Input: part model. Units: mm. Frame: model coordinates. A direction names the side the tool comes from. Round coordinates to 2 decimals unless told otherwise and drop trailing zeros. Loops run counter-clockwise (first coordinate to the right, second up) from the corner with the lowest first, then second, coordinate; pieces in that order, holes last. Notation, with made-up numbers: M 43.25,-12 L 61.25,-12 A23 cw 61.25,11 Z; hole C 4,11.5 d2. An arc over 180 degrees is marked long. Put each result on its own line as item: value. Start each with the question number.
1) Draft query along Z for faces 1 (the face through (-26, 46, 24.4)), 2 (the face through (-40.5, 28, 16)), 3 (the face through (-35, 28, 2)). Return one class per face: +Z half, -Z half, draft (parallel to the pull), parting line (faces both ways), or undercut.
2) Section B-B on x = -34. Output: boundary loops of the cut face in (y, z), plus the area to 3 significant figures.
3) Pin query (flat end, axial travel): pin 1 (2 mm diameter, centred on y = 39.5, z = 22, fed in from +X); pin 2 (14 mm diameter, centred on x = -18, z = 18, fed in from +Y); pin 3 (5 mm diameter, centred on x = -13, z = 19.5, fed in from +Y). Return the tip coordinate at first contact, or that it passes through.
4) Section D-D on x = -2. Output: boundary loops of the cut face in (y, z), plus the area to 4 significant figures.
5) Line query: probe 1 along Z at (x, y) = (-33, 17); probe 2 along Z at (x, y) = (-16, 53.7); probe 3 along X at (y, z) = (54.5, 16). Output: solid intervals per line, ascending.
6) Section A-A on z = 16. Output: boundary loops of the cut face in (x, y), plus the area to 3 significant figures.
7) Reachability of faces 4 (the face through (1.5, 27, 21)), 5 (the face through (-16, 31, 28)), 6 (the face through (-11.155, 54.014, 25.315)), 7 (the face through (-35, 27, 4)) from +Z, -Z, +X, -X, +Y, -Y: full face, straight path, thin tool, end or side. Return the list, or none.
8) Section C-C on y = 27.5. Output: boundary loops of the cut face in (x, z).
Autodesk Inventor part; units mm, degrees
ref_plane "YZ Plane" through (0, 0, 0) normal (1, 0, 0) x (0, 1, 0)
ref_plane "XZ Plane" through (0, 0, 0) normal (0, 1, 0) x (-1, 0, 0)
ref_plane "XY Plane" through (0, 0, 0) normal (0, 0, 1) x (1, 0, 0)
sketch "Sketch1" plane through (0, 0, 0) normal (0, 1, 0) x (-1, 0, 0)
  line L0 (32, 32) -> (0, 32)
  line L1 (0, 32) -> (0, 0)
  line L2 (0, 0) -> (32, 0)
  line L3 (32, 0) -> (32, 32)
extrude "Extrusion1" add sketch "Sketch1" along normal blind 55
sketch "Sketch2" plane through (0, 55, 0) normal (0, 1, 0) x (1, 0, 0)
  line L0 (-9.6, -9.6) -> (-22.4, -9.6)
  line L1 (-22.4, -9.6) -> (-22.4, -22.4)
  line L2 (-22.4, -22.4) -> (-9.6, -22.4)
  line L3 (-9.6, -22.4) -> (-9.6, -9.6)
  point P0 (0, 0)
extrude "Extrusion2" cut sketch "Sketch2" against normal blind 30
sketch "Sketch3" plane through (-32, 0, 32) normal (0, 0, 1) x (1, 0, 0)
  line L0 (3.5, 49) -> (28.5, 49)
  line L1 (28.5, 49) -> (28.5, 31)
  line L2 (28.5, 31) -> (3.5, 31)
  line L3 (3.5, 31) -> (3.5, 49)
  line L4 (3.5, 49) -> (3.5, 43.25)
  line L5 (3.5, 36.75) -> (3.5, 43.25)
  line L6 (28.5, 49) -> (28.5, 43.25)
  line L7 (28.5, 36.75) -> (28.5, 43.25)
  line L8 (3.5, 43.25) -> (3.5, 36.75)
  line L9 (28.5, 43.25) -> (28.5, 36.75)
  point P0 (32, 0)
extrude "Extrusion3" cut sketch "Sketch3" against normal blind 8.6
sketch "Sketch4" plane through (-32, 0, 23.4) normal (0, 0, 1) x (1, 0, 0)
  line L0 (3.5, 49) -> (28.5, 49)
  line L1 (3.5, 49) -> (3.5, 43.25)
  line L2 (28.5, 31) -> (3.5, 31)
  line L3 (3.5, 36.75) -> (3.5, 31)
  line L4 (3.5, 31) -> (28.5, 31)
  line L5 (28.5, 31) -> (28.5, 36.75)
  line L6 (28.5, 49) -> (28.5, 31)
  line L7 (28.5, 43.25) -> (28.5, 49)
  line L8 (28.5, 49) -> (3.5, 49)
  point P0 (32, 0)
sketch "Sketch5" plane through (-32, 0, 23.4) normal (0, 0, 1) x (1, 0, 0)
  line L0 (3.5, 43.25) -> (8.5, 43.25)
  line L1 (8.5, 43.25) -> (8.5, 36.75)
  line L2 (8.5, 36.75) -> (3.5, 36.75)
  line L3 (3.5, 36.75) -> (3.5, 43.25)
  point P0 (32, 0)
sketch "Sketch6" plane through (-32, 0, 23.4) normal (0, 0, 1) x (1, 0, 0)
  line L0 (28.5, 43.25) -> (23.5, 43.25)
  line L1 (23.5, 43.25) -> (23.5, 36.75)
  line L2 (23.5, 36.75) -> (28.5, 36.75)
  line L3 (28.5, 36.75) -> (28.5, 43.25)
  point P0 (32, 0)
extrude "Extrusion4" cut sketch "Sketch5" against normal blind 2
extrude "Extrusion5" cut sketch "Sketch6" against normal blind 2
sketch "Sketch7" plane through (-32, 0, 23.4) normal (0, 0, 1) x (1, 0, 0)
  line L0 (3.5, 43.25) -> (8.5, 43.25)
  line L1 (3.5, 43.25) -> (3.5, 49)
  line L2 (8.5, 43.25) -> (3.5, 43.25)
  line L3 (3.5, 43.25) -> (3.5, 49)
  line L4 (3.5, 49) -> (8.5, 49)
  line L5 (8.5, 49) -> (8.5, 43.25)
  point P0 (32, 0)
sketch "Sketch8" plane through (-32, 0, 23.4) normal (0, 0, 1) x (1, 0, 0)
  line L0 (8.5, 36.75) -> (3.5, 36.75)
  line L1 (28.5, 31) -> (3.5, 31)
  line L2 (8.5, 36.75) -> (3.5, 36.75)
  line L3 (3.5, 36.75) -> (3.5, 31)
  line L4 (3.5, 31) -> (8.5, 31)
  line L5 (8.5, 31) -> (8.5, 36.75)
  point P0 (32, 0)
sketch "Sketch9" plane through (-32, 0, 23.4) normal (0, 0, 1) x (1, 0, 0)
  line L0 (28.5, 36.75) -> (23.5, 36.75)
  line L1 (28.5, 31) -> (3.5, 31)
  line L2 (23.5, 36.75) -> (28.5, 36.75)
  line L3 (28.5, 36.75) -> (28.5, 31)
  line L4 (28.5, 31) -> (23.5, 31)
  line L5 (23.5, 31) -> (23.5, 36.75)
  point P0 (32, 0)
sketch "Sketch10" plane through (-32, 0, 23.4) normal (0, 0, 1) x (1, 0, 0)
  line L0 (23.5, 43.25) -> (28.5, 43.25)
  line L1 (28.5, 49) -> (28.5, 43.25)
  line L2 (23.5, 43.25) -> (28.5, 43.25)
  line L3 (28.5, 43.25) -> (28.5, 49)
  line L4 (28.5, 49) -> (23.5, 49)
  line L5 (23.5, 49) -> (23.5, 43.25)
  point P0 (32, 0)
extrude "Extrusion6" add sketch "Sketch7" along normal blind 1
extrude "Extrusion7" add sketch "Sketch8" along normal blind 1
extrude "Extrusion8" add sketch "Sketch9" along normal blind 1
extrude "Extrusion9" add sketch "Sketch10" along normal blind 1
sketch "Sketch11" plane through (-32, 0, 24.4) normal (0, 0, 1) x (1, 0, 0)
  line L0 (23.5, 43.25) -> (28.5, 43.25)
  line L1 (23.5, 43.25) -> (25, 43.25)
  line L2 (25, 43.25) -> (25, 44.25)
  line L3 (25, 44.25) -> (23.5, 44.25)
  line L4 (23.5, 44.25) -> (23.5, 43.25)
  point P0 (32, 0)
extrude "Extrusion10" cut sketch "Sketch11" against normal blind 1
sketch "Sketch12" plane through (-32, 0, 23.4) normal (0, 0, 1) x (1, 0, 0)
  line L0 (8.5, 49) -> (8.5, 43.25)
  line L1 (23.5, 31) -> (8.5, 31)
  line L2 (23.5, 49) -> (23.5, 44.25)
  point P0 (32, 0)
sketch "Sketch13" plane through (-32, 0, 23.4) normal (0, 0, 1) x (1, 0, 0)
  point P0 (32, 0)
sketch "Sketch14" plane through (-32, 0, 23.4) normal (0, 0, 1) x (1, 0, 0)
  line L0 (23.5, 44.25) -> (23.5, 49)
  line L1 (23.5, 49) -> (17.5, 49)
  line L2 (14.5, 43) -> (17.5, 43)
  line L3 (17.5, 38) -> (18, 38)
  line L4 (18, 38) -> (18, 43)
  line L5 (18, 43) -> (14, 43)
  line L6 (14, 43) -> (14, 38)
  line L7 (14, 38) -> (14.5, 38)
  line L8 (14.5, 38) -> (14.5, 42)
  line L9 (3.5, 43.25) -> (8.5, 43.25)
  line L10 (14.5, 42) -> (14.5, 42.5)
  line L11 (14.5, 42.5) -> (17.5, 42.5)
  line L12 (17.5, 42.5) -> (17.5, 38)
  point P0 (32, 0)
extrude "Extrusion11" add sketch "Sketch14" along normal blind 1
sketch "Sketch15" plane through (-32, 0, 23.4) normal (0, 0, 1) x (1, 0, 0)
  line L0 (14.5, 42.5) -> (14.5, 38)
  line L1 (14.5, 42.5) -> (17.5, 42.5)
  line L2 (17.5, 42.5) -> (17.5, 39.5)
  line L3 (17.5, 39.5) -> (14.5, 39.5)
  line L4 (14.5, 39.5) -> (14.5, 42.5)
  point P0 (32, 0)
extrude "Extrusion12" cut sketch "Sketch15" against normal blind 7.1
sketch "Sketch16" plane through (-32, 0, 32) normal (0, 0, 1) x (1, 0, 0)
  point P0 (32, 0)
sketch "Sketch17" plane through (0, 0, 32) normal (1, 0, 0) x (0, 0, -1)
  line L0 (2, 46) -> (20, 46)
  line L1 (20, 46) -> (20, 8)
  line L2 (20, 8) -> (2, 8)
  line L3 (2, 8) -> (2, 46)
  point P0 (32, 0)
extrude "Extrusion13" cut sketch "Sketch17" against normal blind 1.5
sketch "Sketch18" plane through (-1.5, 0, 32) normal (1, 0, 0) x (0, 0, -1)
  line L0 (20, 38.5) -> (14, 38.5)
  line L1 (14, 38.5) -> (14, 46)
  line L2 (14, 46) -> (20, 46)
  line L3 (20, 46) -> (20, 38.5)
  point P0 (32, 0)
extrude "Extrusion14" cut sketch "Sketch18" against normal blind 8.1
sketch "Sketch19" plane through (0, 55, 0) normal (0, 1, 0) x (1, 0, 0)
  circle A0 centre (-16, -16) radius 10.5
  point P0 (0, 0)
sketch "Sketch20" plane through (0, 55, 0) normal (0, 1, 0) x (1, 0, 0)
  point P0 (0, 0)
extrude "Extrusion15" cut sketch "Sketch19" against normal blind 2
sketch "Sketch21" plane through (-32, 0, 0) normal (-1, 0, 0) x (0, 0, 1)
  line L0 (32, 0) -> (32, 55)
  line L1 (0, 0) -> (32, 0)
  line L2 (32, 0) -> (32, 55)
  line L3 (32, 55) -> (0, 55)
  line L4 (0, 55) -> (0, 0)
extrude "Extrusion16" add sketch "Sketch21" along normal blind 8.5
sketch "Sketch22" plane through (-40.5, 0, 0) normal (-1, 0, 0) x (0, 0, 1)
  line L0 (2, 3) -> (4, 3)
  line L1 (4, 3) -> (4, 52)
  line L2 (4, 52) -> (2, 52)
  line L3 (2, 52) -> (2, 3)
  line L4 (23, 3) -> (25, 3)
  line L5 (25, 3) -> (25, 52)
  line L6 (25, 52) -> (23, 52)
  line L7 (23, 52) -> (23, 3)
  point P0 (0, 0)
extrude "Extrusion17" cut sketch "Sketch22" against normal blind 11
sketch "Sketch23" plane through (0, 0, 32) normal (1, 0, 0) x (0, 0, -1)
  line L0 (0, 0) -> (32, 0)
  line L1 (0, 55) -> (32, 55)
  line L2 (0, 0) -> (32, 0)
  line L3 (32, 0) -> (32, 55)
  line L4 (32, 55) -> (0, 55)
  line L5 (0, 55) -> (0, 0)
sketch "Sketch24" plane through (0, 0, 32) normal (1, 0, 0) x (0, 0, -1)
  line L0 (20, 8) -> (2, 8)
  line L1 (20, 46) -> (20, 8)
  line L2 (2, 8) -> (20, 8)
  line L3 (20, 8) -> (20, 46)
  line L4 (20, 46) -> (2, 46)
  line L5 (2, 46) -> (2, 8)
  point P0 (32, 0)
extrude "Extrusion18" add sketch "Sketch23" along normal blind 3
extrude "Extrusion19" cut sketch "Sketch24" along normal blind 3
sketch "Sketch25" plane through (-1.5, 0, 32) normal (1, 0, 0) x (0, 0, -1)
  line L0 (2, 8) -> (2, 46)
  line L1 (20, 8) -> (2, 8)
  line L2 (2, 8) -> (20, 8)
  line L3 (20, 38.5) -> (20, 8)
  line L4 (20, 8) -> (20, 38.5)
  line L5 (14, 38.5) -> (14, 46)
  line L6 (20, 38.5) -> (14, 38.5)
  line L7 (14, 38.5) -> (14, 46)
  line L8 (14, 46) -> (2, 46)
  point P0 (32, 0)
extrude "Extrusion20" add sketch "Sketch25" along normal blind 3
properties part number "Cuvette Holder v2_3DPrint"
Geometry results:
1. face 1: +Z half
1. face 2: draft
1. face 3: undercut
2. outline: M 0,0 L 55,0 L 55,32 L 0,32 Z; hole M 3,2 L 52,2 L 52,4 L 3,4 Z; hole M 3,23 L 52,23 L 52,25 L 3,25 Z
2. area: 1,560 mm²
3. pin 1: stops at x = 1.5
3. pin 2: stops at y = 53
3. pin 3: stops at y = 25
4. outline: M 0,0 L 55,0 L 55,32 L 0,32 Z; hole M 38.5,12 L 46,12 L 46,18 L 38.5,18 Z
4. area: 1,715 mm²
5. probe 1: z = 0 to 2, 4 to 23, 25 to 32
5. probe 2: z = 0 to 5.5, 26.5 to 32
5. probe 3: x = -40.5 to -26.5, -5.5 to 3
6. outline: M -40.5,0 L 3,0 L 3,8 L 1.5,8 L 1.5,38.5 L -9.6,38.5 L -9.6,25 L -22.4,25 L -22.4,53 L -26.5,53 L -26.5,55 L -40.5,55 Z; M -9.6,46 L 3,46 L 3,55 L -5.5,55 L -5.5,53 L -9.6,53 Z
6. area: 1,850 mm²
7. face 4: +X
7. face 5: +Z
7. face 6: +Y
7. face 7: -X
8. outline: M -40.5,0 L 3,0 L 3,12 L 1.5,12 L 1.5,30 L 3,30 L 3,32 L -40.5,32 L -40.5,25 L -29.5,25 L -29.5,23 L -40.5,23 L -40.5,4 L -29.5,4 L -29.5,2 L -40.5,2 Z; hole M -22.4,9.6 L -9.6,9.6 L -9.6,22.4 L -22.4,22.4 Z
